The listing builds one solid part. Answer for the finished solid, in the listing's coordinates (mm). Coordinates: 2 decimals unless noted, no trailing zeros. Write each loop counter-clockwise with the first axis right and the second up, starting at its lowest first coordinate (ties: lowest second). Pieces come first, ordered by that corner, then holes.
```python
from build123d import *

# Parameters (mm, degrees)
BASE_FLANGE1_DEPTH = 1
FILLET1_R          = 3
SKETCH2_R          = 2.5
CUT_EXTRUDE1_DEPTH = 10


# Sheet-metal steps are written as plain solids
with BuildPart() as part:
    # Sketch1 → Base-Flange1 (new body)
    with BuildSketch(Plane.XY):
        Polygon((0, 0), (0, 243.736706628), (412, 481.605017534), (412, 586.417185402), (-91, 296.01), (-91, 0), align=None)
    extrude(amount=-BASE_FLANGE1_DEPTH)

    # Fillet1
    fillet1_edges = [part.edges().sort_by_distance(p)[0] for p in [
        (-91, 0, -0.5),
        (-91, 296.01, -0.5),
        (412, 586.417185402, -0.5),
        (412, 481.605017534, -0.5),
        (0, 243.736706628, -0.5),
        (0, 0, -0.5),
    ]]
    fillet(fillet1_edges, radius=FILLET1_R)

    # Sketch2 → Cut-Extrude1 (cut)
    with BuildSketch(Plane(origin=(0, 0, -1), x_dir=(-1, 0, 0), z_dir=(0, 0, -1))):
        with Locations((-382, 562.168474096)):
            Circle(SKETCH2_R)
        with Locations((-240.404846481, 480.418474096)):
            Circle(SKETCH2_R)
        with Locations((-98.809692962, 398.668474096)):
            Circle(SKETCH2_R)
        with Locations((42.785460556, 316.918474096)):
            Circle(SKETCH2_R)
        with Locations((-382, 471.212712688)):
            Circle(SKETCH2_R)
        with Locations((-267.6846467, 405.212712688)):
            Circle(SKETCH2_R)
        with Locations((-153.369293401, 339.212712688)):
            Circle(SKETCH2_R)
        with Locations((-39.053940101, 273.212712688)):
            Circle(SKETCH2_R)
        with Locations((85, 30)):
            Circle(SKETCH2_R)
        with Locations((6, 40)):
            Circle(SKETCH2_R)
        with Locations((85, 140)):
            Circle(SKETCH2_R)
        with Locations((85, 250)):
            Circle(SKETCH2_R)
        with Locations((6, 205)):
            Circle(SKETCH2_R)
    extrude(amount=-CUT_EXTRUDE1_DEPTH, mode=Mode.SUBTRACT)


solid = part.part
```
(1) Find the intervals of material crossed by probe 1 along X at (y, z) = (205, -0.3); probe 2 along X at (y, z) = (140, -0.5); probe 3 along X at (y, z) = (87.5, -0.9), in increasing order.
(2) Section A-A, the plane z = -0.8 is taken. State how many separate pieces and enclosed holes the cut face has, plus the area to 3 significant figures.
(3) Section C-C, the plane x = 322.5 is taken. Write down the section's boundary in (y, z).
(4) Section B-B, the plane y = 62 is taken. Write down the section's boundary in (x, z), plus the area to 3 significant figures.
Solution:
1. probe 1: x = -91 to -8.5, -3.5 to 0
1. probe 2: x = -91 to -87.5, -82.5 to 0
1. probe 3: x = -91 to 0
2. separate pieces: 1
2. enclosed holes: 13
2. area: 72,200 mm2
3. outline: (429.93, -1) - (534.74, -1) - (534.74, 0) - (429.93, 0) - close
4. outline: (-91, -1) - (0, -1) - (0, 0) - (-91, 0) - close
4. area: 91.0 mm2
